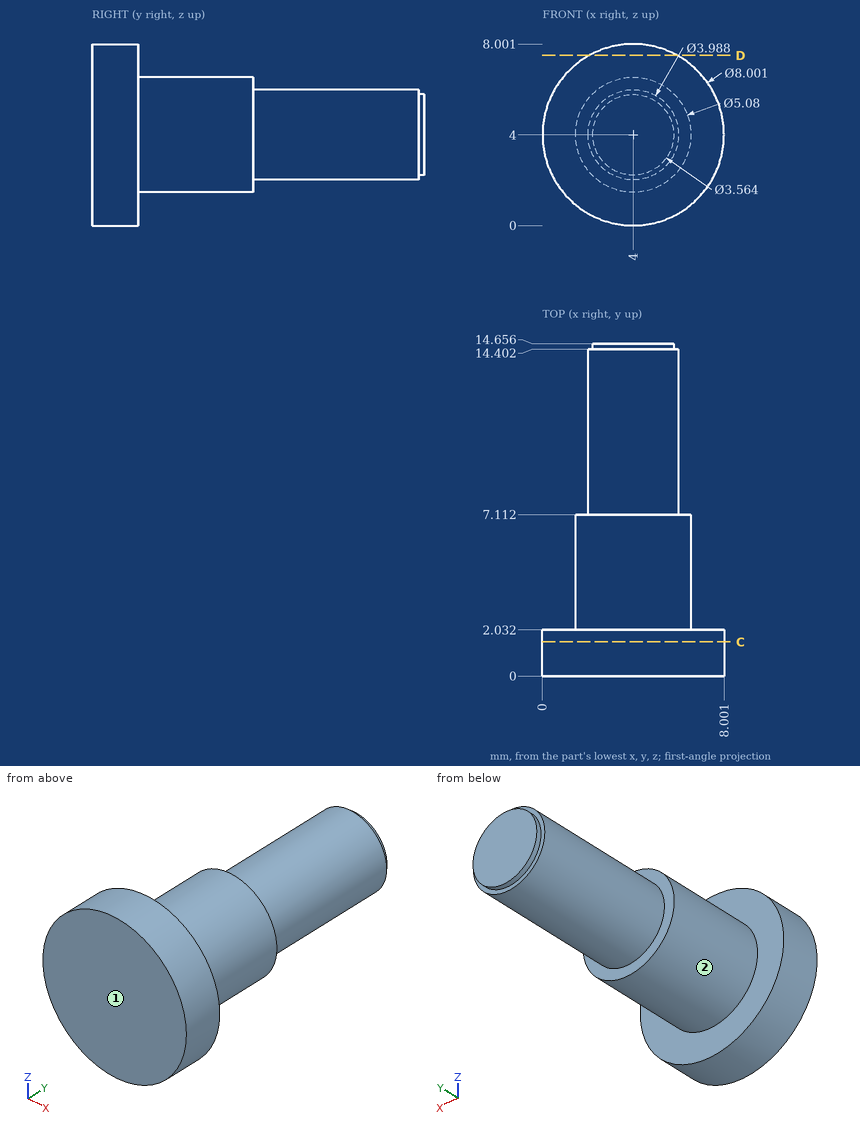
Job drawing, mm, ordinate dimensions from the low corner. One solid piece. A direction names the side the tool comes from. Round coordinates to 2 decimals unless told otherwise and drop trailing zeros. Loops run counter-clockwise (first coordinate to the right, second up) from the corner with the lowest first, then second, coordinate; pieces in that order, holes last.
Item 1: Cut at C-C, the plane y = 1.5. Give the cut face in (x, z), then the cut area to 3 significant figures.
Item 2: 3-axis set-ups, long thin cutter, end or side, ignore diameter. For the marked faces 1 and 2: which of +Z, -Z, +X, -X, +Y, -Y reach the whole face in a straight line?
Item 3: Cut at D-D, the plane z = 7.5. Give the cut face in (x, y).
Item 4: Drill centre lines: line 1 (Y direction, x = 2.75, z = 0.5); line 2 (Z direction, x = 2.5, y = 2.25); line 3 (Z direction, x = 5, y = 2.5) (1 decimal). Where is each one in solid material? Low to high.
Item 5: Drop flat-ended pins along their axis: P1, Ø4, axis at y = 12, z = 3.5, coming from the -X side; P2, Ø1, axis at x = 1, z = 3, coming from the +Y side; P3, Ø1.5, axis at x = 6, y = 12, coming from the -Z side (1 decimal). Give the stop position or say it passes through.
A:
1. outline: circle Ø8 at (4, 4)
1. area: 50.3 mm2
2. face 1: +Z, -Z, +X, -X, -Y
2. face 2: +Y
3. outline: (2.06, 0) - (5.94, 0) - (5.94, 2.03) - (2.06, 2.03) - close
4. line 1: y = 0 to 2.03
4. line 2: z = 1.95 to 6.05
4. line 3: z = 1.7 to 6.3
5. P1: stops at x = 2.01
5. P2: stops at y = 2.03
5. P3: stops at z = 2.4
